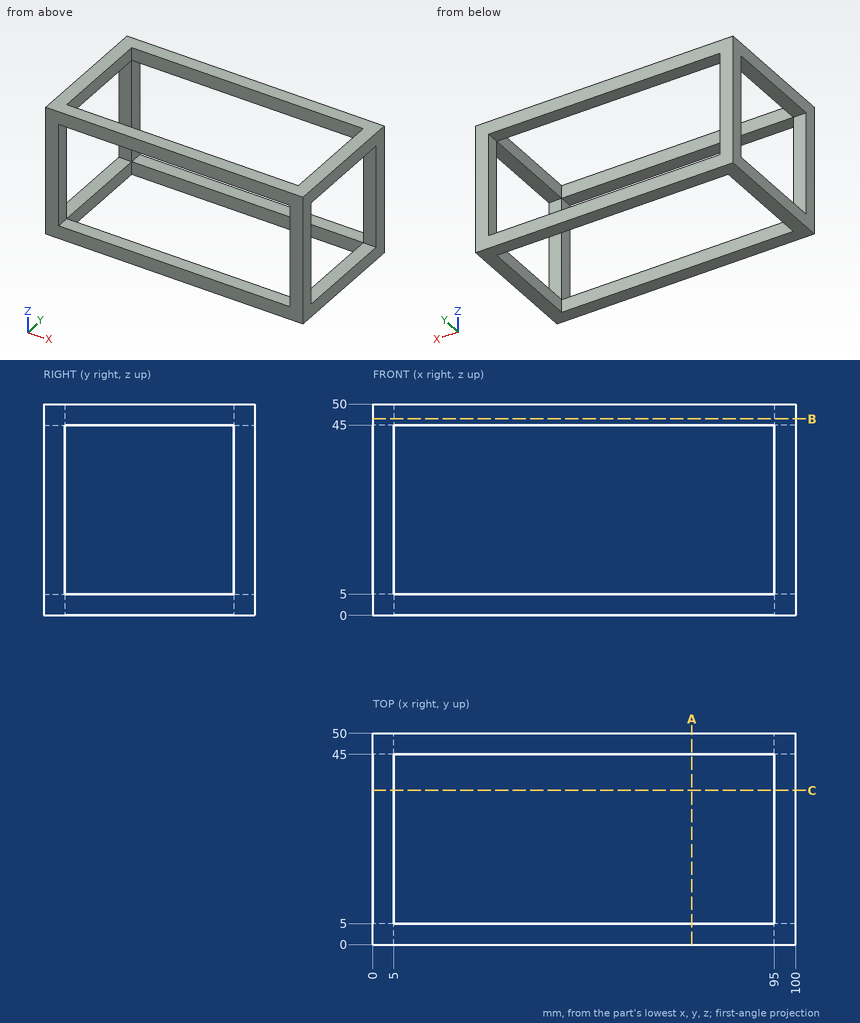
Geometry check sheet. Reference: drawing and pictorial views, mm from the part's lowest x, y, z. Round coordinates to 2 decimals unless told otherwise and drop trailing zeros. Order: outer loops, then holes, each group sorted by start corner. A loop starts at its lowest first (then second) coordinate and runs counter-clockwise, first axis right, second up. Notation, with made-up numbers: (81, -3.75) - (119, -3.75) arc R22 cw to (119, 2.25) - close; hole circle Ø7 at (44.25, -24). An arc over 180 degrees is marked (long way). One line per question, with ' | ' between items. Start each with the question number.
(1) Depth check by flat-ended pin: pin 1 Ø2.5 at (y, z) = (34.5, 2.5) entering from -X. Enter the tip coordinate at first touch or a pass-through.
(2) Sectioned sample at B-B on z = 46.5. Record the cut outline in (x, y), and give its area (3 significant figures).
(3) Thickness scan on L1, parallel to Y at x = 96.5, z = 31; L2, parallel to X at y = 19.5, z = 47.5. Record the ranges inside material, lowest first. Write a range as [from, to].
(4) Sectioned sample at A-A on x = 75.5. Record the cut outline in (y, z).
(5) Sectioned sample at C-C on y = 36.5. Record the cut outline in (x, z).
Conclusion:
1) pin 1: stops at x = 0
2) outline: (0, 0) - (100, 0) - (100, 50) - (0, 50) - close; hole (5, 5) - (95, 5) - (95, 45) - (5, 45) - close | area: 1,400 mm2
3) L1: y = [0, 5], [45, 50] | L2: x = [0, 5], [95, 100]
4) outline: (0, 0) - (5, 0) - (5, 5) - (0, 5) - close; (0, 45) - (5, 45) - (5, 50) - (0, 50) - close; (45, 0) - (50, 0) - (50, 5) - (45, 5) - close; (45, 45) - (50, 45) - (50, 50) - (45, 50) - close
5) outline: (0, 0) - (5, 0) - (5, 5) - (0, 5) - close; (0, 45) - (5, 45) - (5, 50) - (0, 50) - close; (95, 0) - (100, 0) - (100, 5) - (95, 5) - close; (95, 45) - (100, 45) - (100, 50) - (95, 50) - close
